Read the model definition and answer for the solid it produces. Units are mm, in the model's axes. A direction names the side the tool comes from. Give positions to 0.01 mm unless a question says otherwise; leave off trailing zeros. Order: outer loops, then holes, each group sorted by start corner. A loop starts at its lowest first (then second) coordinate and runs counter-clockwise, first axis right, second up. Notation, with made-up numbers: M 40,-18 L 93,-18 A24 ccw 93,5 Z; hole C 73.5,-34.5 d7. An arc over 180 degrees is marked long. One line per item, written item: value.
from build123d import *

# Parameters (mm, degrees)
SKETCH1_R           = 35
SKETCH1_R_2         = 17.5
BOSS_EXTRUDE1_DEPTH = 50
CUT_EXTRUDE1_START  = -14
CUT_EXTRUDE1_DEPTH  = 14


with BuildPart() as part:
    # Sketch1 → Boss-Extrude1 (new body)
    with BuildSketch(Plane(origin=(0, 0, 0), x_dir=(1, 0, 0), z_dir=(0, 1, 0))):
        with Locations(Location((0, 0, 0), (0, 0, 270))):
            Circle(SKETCH1_R)
        with Locations(Location((0, 0, 0), (0, 0, 270))):
            Circle(SKETCH1_R_2, mode=Mode.SUBTRACT)
    extrude(amount=BOSS_EXTRUDE1_DEPTH)

    # Sketch2 → Cut-Extrude1 (cut)
    with BuildSketch(Plane(origin=(0, 50, 0), x_dir=(1, 0, 0), z_dir=(0, 1, 0)).offset(CUT_EXTRUDE1_START)):
        with BuildLine():
            Line((15.155444566, -8.75), (30.310889132, -17.5))
            ThreePointArc((30.310889132, -17.5), (0, -35), (-30.310889132, -17.5))
            Line((-30.310889132, -17.5), (-15.155444566, -8.75))
            ThreePointArc((-15.155444566, -8.75), (0, -17.5), (15.155444566, -8.75))
        make_face()
    cut_extrude1 = extrude(amount=CUT_EXTRUDE1_DEPTH, mode=Mode.SUBTRACT)

    # Mirror1: Cut-Extrude1 across plane
    add(cut_extrude1.mirror(Plane.XY), mode=Mode.SUBTRACT)


solid = part.part
1) Find section A-A, the plane z = 0. Write down the section's boundary in (x, y), plus the area to 3 significant figures.
Reported:
outline: M -35,0 L -17.5,0 L -17.5,50 L -35,50 Z; M 17.5,0 L 35,0 L 35,50 L 17.5,50 Z
area: 1,750 mm^2
2) Determine the mould class of faces 4 (the face through (0, 36, -22)), 5 (the face through (-31.05, 19.09, 16.15)), 6 (the face through (25, 50, 0)) for opening direction X: +X half, -X half, draft (parallel to the pull), parting line (faces both ways), or undercut.
Reported:
face 4: undercut
face 5: parting line
face 6: draft
3) Find section B-B, the plane x = 0. Write down the section's boundary in (y, z).
Reported:
outline: M 0,-35 L 36,-35 L 36,-17.5 L 0,-17.5 Z; M 0,17.5 L 36,17.5 L 36,35 L 0,35 Z
4) Consider probe 1 along X at (y, z) = (16, 0); probe 2 along Y at (x, z) = (-4.5, -24); probe 3 along X at (y, z) = (46.5, 7). Determine where each line is inside the solid, lowest interval first.
Reported:
probe 1: x = -35 to -17.5, 17.5 to 35
probe 2: y = 0 to 36
probe 3: x = -34.29 to -16.04, 16.04 to 34.29
5) Find section C-C, the plane y = 12.5. Write down the section's boundary in (x, z).
Reported:
outline: C 0,0 d70; hole C 0,0 d35
6) Find section D-D, the plane x = 19. Write down the section's boundary in (y, z).
Reported:
outline: M 0,-29.39 L 36,-29.39 L 36,-10.97 L 50,-10.97 L 50,10.97 L 36,10.97 L 36,29.39 L 0,29.39 Z
7) Which of the six approach directions +Z, -Z, +X, -X, +Y, -Y give full straight-line access (tool end or side, diameter ignored) to faces 1 (the face through (-15.526, 19.094, 8.075)), 2 (the face through (-22.839, 42.902, 13.186)), 3 (the face through (-22.839, 42.902, -13.186))?
Reported:
face 1: +Y, -Y
face 2: +Z, +Y
face 3: -Z, +Y
8) Each of these flat-tipped pins is pushed along its axis until it touches: pin 1 Ø8 at (x, z) = (4, 17.5) entering from -Y; pin 2 Ø8 at (x, y) = (12, 29.5) entering from +Z; pin 3 Ø21 at (x, z) = (-2, -19.5) entering from +Y; pin 4 Ø5 at (y, z) = (42.5, -10) entering from +X. Where does it stop, or does it pass through?
Reported:
pin 1: stops at y = 0
pin 2: stops at z = 34.07
pin 3: stops at y = 36
pin 4: stops at x = 34.19
